Can you work these out from the model? Positions are in its coordinate system, mm. A direction names the side the tool comes from. Round coordinates to 2 decimals unless told otherwise and drop trailing zeros. Loops run counter-clockwise (first coordinate to the right, second up) from the corner with the lowest first, then second, coordinate; pieces in that order, holes last. Notation, with made-up numbers: M -24,56 L 1,56 A24 cw 1,68 Z; hole C -21.5,88 d3. An arc over 180 degrees is marked long. Return JSON: item names as keys, results as strings.
```python
from build123d import *

# Parameters (mm, degrees)
F0_W     = 85.1215273142
F0_H     = 42.9548472166
F1_DEPTH = 7.62
F2_R     = 7.62
F4_DEPTH = 25.4
F5_DEPTH = 25.4


with BuildPart() as f1:
    # F0 (on Top) → F1 (new body)
    with BuildSketch(Plane.XY):
        Rectangle(F0_W, F0_H)
    extrude(amount=F1_DEPTH)

    # F2
    f2_edges = [f1.edges().sort_by_distance(p)[0] for p in [
        (-42.560764, 21.477424, 3.81),
        (42.560764, 21.477424, 3.81),
    ]]
    fillet(f2_edges, radius=F2_R)

    # F3 (on face) → F4 (join)
    with BuildSketch(Plane.XY.offset(7.62)):
        with BuildLine():
            Line((12.9238776863, 21.4774236083), (11.2444977121, 21.4774236083))
            ThreePointArc((11.2444977121, 21.4774236083), (0, 10.2329258962), (-11.2444977121, 21.4774236083))
            Line((-11.2444977121, 21.4774236083), (-12.9238776863, 21.4774236083))
            Line((-12.9238776863, 21.4774236083), (-12.9238776863, 0))
            ThreePointArc((-12.9238776863, 0), (-14.282709623, -3.2805104906), (-17.5632201135, -4.6393424273))
            Line((-17.5632201135, -4.6393424273), (-17.5632201135, -21.4774236083))
            Line((-17.5632201135, -21.4774236083), (-10.9355887398, -21.4774236083))
            Line((-10.9355887398, -21.4774236083), (-10.9355887398, -13.5037954897))
            Line((-10.9355887398, -13.5037954897), (-3.6451956257, -13.5037954897))
            Line((-3.6451956257, -13.5037954897), (3.6451956257, -13.5037954897))
            Line((3.6451956257, -13.5037954897), (10.9355887398, -13.5037954897))
            Line((10.9355887398, -13.5037954897), (10.9355887398, -21.4774236083))
            Line((10.9355887398, -21.4774236083), (17.5632201135, -21.4774236083))
            Line((17.5632201135, -21.4774236083), (17.5632201135, -4.6393424273))
            ThreePointArc((17.5632201135, -4.6393424273), (14.282709623, -3.2805104906), (12.9238776863, 0))
            Line((12.9238776863, 0), (12.9238776863, 21.4774236083))
        make_face()
    extrude(amount=F4_DEPTH)

    # F5 (cut): a face of the model
    f5_faces = [f1.faces().sort_by_distance(p)[0] for p in [
        (0, 16.7051105591, 7.62),
    ]]
    extrude(f5_faces, amount=-F5_DEPTH, mode=Mode.SUBTRACT)


solid = f1.part
```
Q1. Suppose I cut it at D-D, the plane x = -21.5. Please give me the cut outline in (y, z), plus the area to 3 significant figures.
Results:
{"outline": "M -21.48,0 L 21.48,0 L 21.48,7.62 L -21.48,7.62 Z", "area": "327 mm2"}
Q2. Thinking about a two-plate mould opening in X: for faces 5 (the flat face through (0, -17, 7.62)), 6 (the flat face through (-28, 0, 7.62)), 7 (the cylindrical face through (0.247, 10.236, 16.741)), 8 (the cylindrical face through (40.388, 19.186, 3.863)), which applies, pulls with the +X half, pulls with the -X half, needs draft (parallel to the pull), parting line crosses it, or undercut?
Results:
{"face 5": "undercut", "face 6": "needs draft", "face 7": "undercut", "face 8": "pulls with the +X half"}
Q3. On a 3-axis mill with a long thin cutter (end or side, diameter ignored), from which of +Z, -Z, +X, -X, +Y, -Y can I reach the whole of each face in a straight line? I mean faces 1 (the flat face through (10.936, -17, 20)), 2 (the flat face through (17.563, -13, 20)), 3 (the cylindrical face through (-14.247, -3.244, 20.142)), 4 (the flat face through (12.924, 11, 20)). Say none if no direction works.
Results:
{"face 1": "+Z, -Y", "face 2": "+Z, +X, +Y, -Y", "face 3": "+Z, -X, +Y", "face 4": "+Z, +X, +Y"}
Q4. Suppose I cut it at B-B, the plane x = 0. Please give me the cut outline in (y, z).
Results:
{"outline": "M -21.48,0 L 10.23,0 L 10.23,33.02 L -13.5,33.02 L -13.5,7.62 L -21.48,7.62 Z"}
Q5. Suppose I cut it at A-A, the plane z = 10. Please give me the cut outline in (x, y), plus the area to 3 significant figures.
Results:
{"outline": "M -17.56,-21.48 L -10.94,-21.48 L -10.94,-13.5 L 10.94,-13.5 L 10.94,-21.48 L 17.56,-21.48 L 17.56,-4.64 A4.64 cw 12.92,0 L 12.92,21.48 L 11.24,21.48 A11.24 cw -11.24,21.48 L -12.92,21.48 L -12.92,0 A4.64 cw -17.56,-4.64 Z", "area": "903 mm2"}
Q6. I'm going to push flat-ended pins straight in: pin 1 Ø9 at (x, y) = (22, 7) entering from +Z; pin 2 Ø6.5 at (y, z) = (13, 22) entering from -X; pin 3 Ø9 at (y, z) = (-17, 22) entering from -X; pin 4 Ø6.5 at (x, y) = (-0.5, -16) entering from +Z. Where does each tip first touch, or does it pass through?
Results:
{"pin 1": "stops at z = 7.62", "pin 2": "stops at x = -12.92", "pin 3": "stops at x = -17.56", "pin 4": "stops at z = 33.02"}
Q7. If I drill on line 1 along X through (y, z) = (-16.5, 20); line 2 along Z through (x, y) = (34.5, -6); line 3 along X through (y, z) = (-12.5, 11.5), over which ranges is the centre line in solid material (lowest first)?
Results:
{"line 1": "x = -17.56 to -10.94, 10.94 to 17.56", "line 2": "z = 0 to 7.62", "line 3": "x = -17.56 to 17.56"}
Q8. Suppose I cut it at C-C, the plane y = -3. Please give me the cut outline in (x, z), plus the area to 3 significant figures.
Results:
{"outline": "M -42.56,0 L 42.56,0 L 42.56,7.62 L 14.02,7.62 L 14.02,33.02 L -14.02,33.02 L -14.02,7.62 L -42.56,7.62 Z", "area": "1,360 mm2"}
